from build123d import *

# Parameters (mm, degrees)
SKETCH1_W                                         = 355.6
SKETCH1_H                                         = 482.6
EXTRUDE1_DEPTH                                    = 7.9375
F_5_16_CLEARANCE_HOLE1_D                          = 8.72998
F_5_16_CLEARANCE_HOLE1_DEPTH                      = 7.9375
CSK_FOR_5_16_FLAT_HEAD_SOCKET_CAP_SC_2_COUNT      = 2
CSK_FOR_5_16_FLAT_HEAD_SOCKET_CAP_SC_2_PITCH      = 405.637419891
CSK_FOR_5_16_FLAT_HEAD_SOCKET_CAP_SC_3_COUNT      = 2
CSK_FOR_5_16_FLAT_HEAD_SOCKET_CAP_SC_3_PITCH      = 101.6
CSK_FOR_5_16_FLAT_HEAD_SOCKET_CAP_SC_4_COUNT      = 2
CSK_FOR_5_16_FLAT_HEAD_SOCKET_CAP_SC_4_PITCH      = 416.444177142
CSK_FOR_6_FLAT_HEAD_SOCKET_CAP_SCREW1_D           = 3.6576
CSK_FOR_6_FLAT_HEAD_SOCKET_CAP_SCREW1_DEPTH       = 7.938008
CSK_FOR_6_FLAT_HEAD_SOCKET_CAP_SCREW1_CSINK_D     = 8.6809834
CSK_FOR_6_FLAT_HEAD_SOCKET_CAP_SCREW1_CSINK_ANGLE = 82
CSK_FOR_6_FLAT_HEAD_SOCKET_CAP_SCREW1_TIP         = 1.0988539


with BuildPart() as part:
    # Sketch1 → Extrude1 (new body)
    with BuildSketch(Plane.XY):
        Rectangle(SKETCH1_W, SKETCH1_H)
    extrude(amount=EXTRUDE1_DEPTH)

    # 5/16 Clearance Hole1
    with Locations(Plane(origin=(0, 0, 0), x_dir=(-1, 0, 0), z_dir=(0, 0, -1))):
        with Locations((59.004201824, 0), (160.604201824, 0)):
            Hole(F_5_16_CLEARANCE_HOLE1_D / 2, depth=F_5_16_CLEARANCE_HOLE1_DEPTH)

    # Sketch12 → CSK for 5/16 Flat Head Socket Cap Screw1 (revolve, cut)
    with BuildSketch(Plane(origin=(51.036073032, 202.818709946, 7.9375), x_dir=(0, -1, 0), z_dir=(1, 0, 0))):
        Polygon((0, 0), (0, 7.9375), (4.2164, 7.9375), (4.2164, 5.241529063), (8.7727917, 0), align=None)
    csk_for_5_16_flat_head_socket_cap_screw1 = revolve(axis=Axis((51.036073032, 202.818709946, 14.2875), (0, 0, -1)), mode=Mode.SUBTRACT)

    # CSK for 5_16 Flat Head Socket Cap Sc 2: CSK for 5/16 Flat Head Socket Cap Screw1 ×2
    with Locations(*[(0, -i * CSK_FOR_5_16_FLAT_HEAD_SOCKET_CAP_SC_2_PITCH, 0) for i in range(1, CSK_FOR_5_16_FLAT_HEAD_SOCKET_CAP_SC_2_COUNT)]):
        add(csk_for_5_16_flat_head_socket_cap_screw1, mode=Mode.SUBTRACT)

    # CSK for 5_16 Flat Head Socket Cap Sc 3: CSK for 5/16 Flat Head Socket Cap Screw1 ×2
    with Locations(*[Vector(-0.999847695, -0.017452406, 0) * (i * CSK_FOR_5_16_FLAT_HEAD_SOCKET_CAP_SC_3_PITCH) for i in range(1, CSK_FOR_5_16_FLAT_HEAD_SOCKET_CAP_SC_3_COUNT)]):
        add(csk_for_5_16_flat_head_socket_cap_screw1, mode=Mode.SUBTRACT)

    # CSK for 5_16 Flat Head Socket Cap Sc 4: CSK for 5/16 Flat Head Socket Cap Screw1 ×2
    with Locations(*[Vector(-0.243933116, -0.969792058, 0) * (i * CSK_FOR_5_16_FLAT_HEAD_SOCKET_CAP_SC_4_PITCH) for i in range(1, CSK_FOR_5_16_FLAT_HEAD_SOCKET_CAP_SC_4_COUNT)]):
        add(csk_for_5_16_flat_head_socket_cap_screw1, mode=Mode.SUBTRACT)

    # CSK for #6 Flat Head Socket Cap Screw1
    with Locations(Plane.XY.offset(7.9375)):
        with Locations((-171.45, -215.9), (171.45, -215.9), (171.45, -161.925), (-171.45, -161.925), (171.45, -107.95), (-171.45, -107.95), (171.45, -53.975), (-171.45, -53.975), (171.45, 0), (-171.45, 0), (171.45, 53.975), (-171.45, 53.975), (171.45, 107.95), (-171.45, 107.95), (171.45, 161.925), (-171.45, 161.925), (171.45, 215.9), (-171.45, 215.9)):
            CounterSinkHole(CSK_FOR_6_FLAT_HEAD_SOCKET_CAP_SCREW1_D / 2, CSK_FOR_6_FLAT_HEAD_SOCKET_CAP_SCREW1_CSINK_D / 2, depth=CSK_FOR_6_FLAT_HEAD_SOCKET_CAP_SCREW1_DEPTH, counter_sink_angle=CSK_FOR_6_FLAT_HEAD_SOCKET_CAP_SCREW1_CSINK_ANGLE)
            with Locations((0, 0, -(CSK_FOR_6_FLAT_HEAD_SOCKET_CAP_SCREW1_DEPTH + CSK_FOR_6_FLAT_HEAD_SOCKET_CAP_SCREW1_TIP / 2))):  # 118° drill point
                Cone(0, CSK_FOR_6_FLAT_HEAD_SOCKET_CAP_SCREW1_D / 2, CSK_FOR_6_FLAT_HEAD_SOCKET_CAP_SCREW1_TIP, mode=Mode.SUBTRACT)


solid = part.part
The model under review builds one solid part; all positions refer to its coordinate system, in mm. Give positions to 0.01 mm unless a question says otherwise; leave off trailing zeros.
1. For P1, Ø4, axis at x = -171.45, y = -53.975, coming from the +Z side; P2, Ø6, axis at x = 171.45, y = 53.975, coming from the +Z side; P3, Ø5, axis at x = -171.45, y = -107.95, coming from the +Z side, all flat-tipped, find the tip position at first contact; note any pin that passes through.
2. Wall thickness on L1, parallel to Y at x = -59, z = 2.5; L2, parallel to X at y = -205, z = 6; L3, parallel to X at y = 202.5, z = 3: over which ranges is each line inside the solid? List them lowest first.
3. Draft analysis for pull direction X (two halves, no side actions). For faces 1 (the flat face through (-2, 3, 0)), 2 (the conical face through (-51.901, 196.752, 3.024)), state which applies: +X half, -X half, draft (parallel to the pull), parting line (faces both ways), or undercut.
Worked answers:
1. P1: stops at z = 5.25
1. P2: stops at z = 6.4
1. P3: stops at z = 5.82
2. L1: y = -241.3 to -4.36, 4.36 to 241.3
2. L2: x = -177.8 to -56.43, -44.67 to 44.29, 57.78 to 177.8
2. L3: x = -177.8 to -54.79, -46.31 to 46.57, 55.51 to 177.8
3. face 1: draft
3. face 2: undercut
